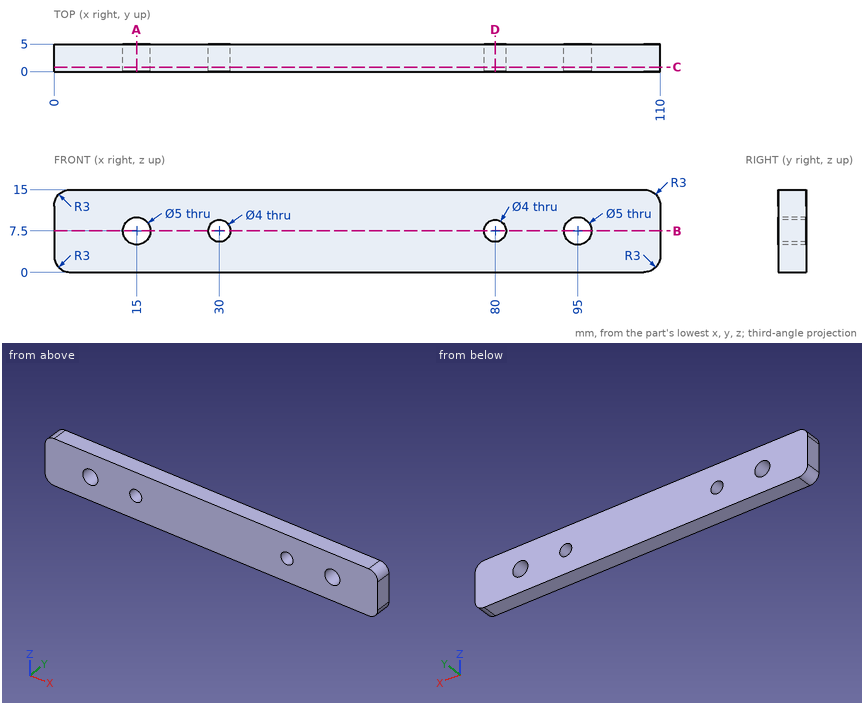
Job drawing, mm, ordinate dimensions from the low corner. One solid piece. Round coordinates to 2 decimals unless told otherwise and drop trailing zeros. Order: outer loops, then holes, each group sorted by start corner. A loop starts at its lowest first (then second) coordinate and runs counter-clockwise, first axis right, second up. Notation, with made-up numbers: M 79,21.25 L 91,21.25 A12 cw 91,32.25 Z; hole C 76,-40 d3. An arc over 180 degrees is marked long. Write each question's results on one line, items separated by ' | '. Start each with the question number.
(1) Saw through at C-C, the plane y = 0.8. Give the cut face in (x, z).
(2) Saw through at A-A, the plane x = 15. Give the cut face in (y, z), then the cut area to 3 significant figures.
(3) Saw through at D-D, the plane x = 80. Give the cut face in (y, z).
(4) Drop a flat-ended pin along its axis: pin 1 (6.5 mm diameter, centred on x = 15, z = 7.5, fed in from +Y). Give the stop position or say it passes through.
(5) Saw through at B-B, the plane z = 7.5. Give the cut face in (x, y).
(6) Probe probe 1 along X at (y, z) = (3.35, 7.5); probe 2 along Z at (x, y) = (30, 1.2); probe 3 along X at (y, z) = (3.2, 6.5). List the from-to ranges inside material, lowest first. Write a range as from..to.
Established:
1) outline: M 0,3 A3 ccw 3,0 L 107,0 A3 ccw 110,3 L 110,12 A3 ccw 107,15 L 3,15 A3 ccw 0,12 Z; hole C 15,7.5 d5; hole C 30,7.5 d4; hole C 80,7.5 d4; hole C 95,7.5 d5
2) outline: M 0,0 L 5,0 L 5,5 L 0,5 Z; M 0,10 L 5,10 L 5,15 L 0,15 Z | area: 50.0 mm^2
3) outline: M 0,0 L 5,0 L 5,5.5 L 0,5.5 Z; M 0,9.5 L 5,9.5 L 5,15 L 0,15 Z
4) pin 1: stops at y = 5
5) outline: M 0,0 L 12.5,0 L 12.5,5 L 0,5 Z; M 17.5,0 L 28,0 L 28,5 L 17.5,5 Z; M 32,0 L 78,0 L 78,5 L 32,5 Z; M 82,0 L 92.5,0 L 92.5,5 L 82,5 Z; M 97.5,0 L 110,0 L 110,5 L 97.5,5 Z
6) probe 1: x = 0..12.5, 17.5..28, 32..78, 82..92.5, 97.5..110 | probe 2: z = 0..5.5, 9.5..15 | probe 3: x = 0..12.71, 17.29..28.27, 31.73..78.27, 81.73..92.71, 97.29..110
